The drawing under review shows one solid part. Ordinate dimensions are in mm from its lowest x, y, z. A direction names the side the tool comes from. Give positions to 0.01 mm unless a question says otherwise; leave off trailing zeros. Order: outer loops, then holes, each group sorted by start corner. A loop starts at its lowest first (then second) coordinate and runs counter-clockwise, first axis right, second up. Notation, with made-up numbers: (49.5, 20) -> (75.5, 20) arc R26 cw to (75.5, 49) -> close; hole circle Ø2 at (-30.5, 5.5). An arc over 180 degrees is marked (long way). One line per item, written item: value. Start each with the question number.
1) Tool access review of the marked faces 5, 6 and 7: name each direction out of +Z, -Z, +X, -X, +Y, -Y from which nothing blocks a thin tool from reaching the whole face with its end or side.
2) Consider section C-C (y = 13.5). State the section outline as (x, z) points.
3) For pin 1 (1 mm diameter, centred on x = 25, z = 20.5, fed in from +Y); pin 2 (6 mm diameter, centred on x = 14.5, z = 20.5, fed in from -Y), all flat-tipped, find the tip position at first contact; note any pin that passes through.
4) Consider section D-D (y = 25). State the section outline as (x, z) points.
5) Consider section A-A (z = 26.5). State the section outline as (x, y) points.
6) The part is to be moulded in two halves that separate along X. For the marked faces 1, 2, 3 and 4, say which applies: released by +X, released by -X, zero draft, split by the parting line, or undercut.
7) Wall thickness on line 1 along Z through (x, y) = (10, 7); line 2 along X through (y, z) = (26.5, 28.5); line 3 along Y through (x, z) = (20, 36): over which ranges is each line inside the solid? List them lowest first. Write a range as from..to.
8) Consider section B-B (x = 15). State the section outline as (y, z) points, plus the area to 3 significant figures.
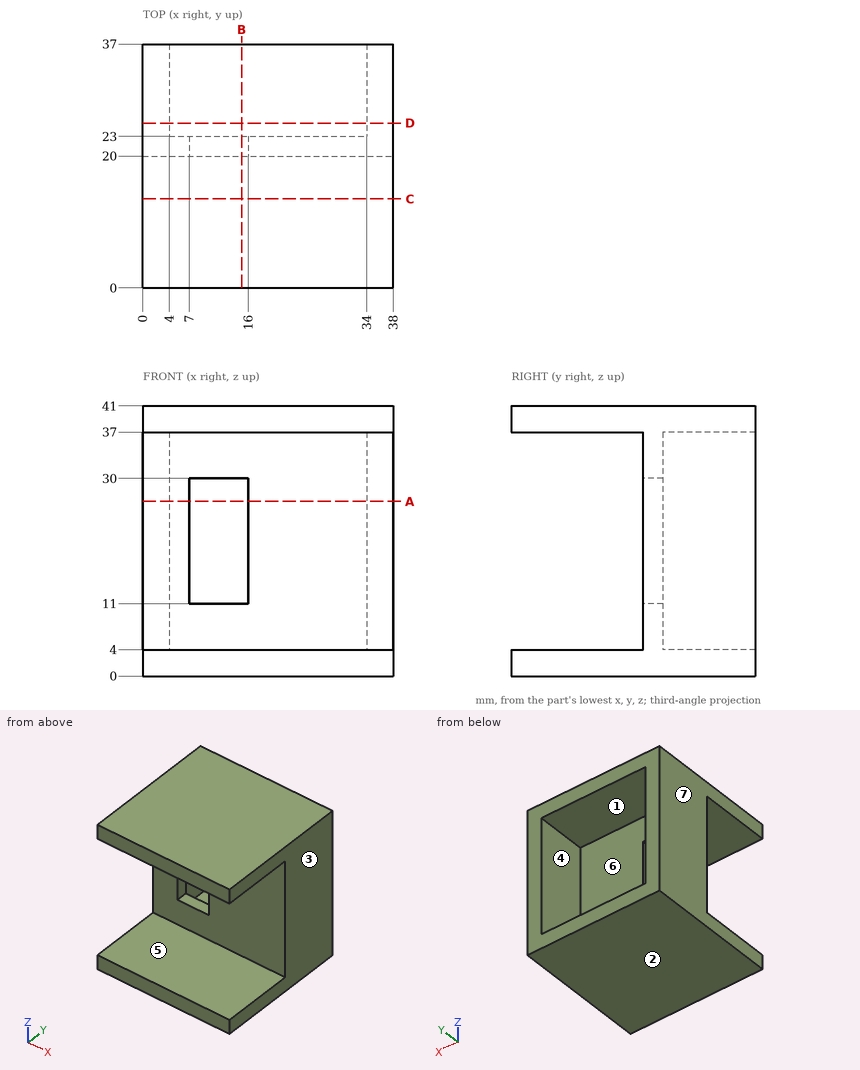
Checked values:
1. face 5: +X, -X, -Y
1. face 6: +Y
1. face 7: +Z, -Z, -X, +Y, -Y
2. outline: (0, 0) -> (38, 0) -> (38, 4) -> (0, 4) -> close; (0, 37) -> (38, 37) -> (38, 41) -> (0, 41) -> close
3. pin 1: stops at y = 23
3. pin 2: stops at y = 20
4. outline: (0, 0) -> (38, 0) -> (38, 41) -> (0, 41) -> close; hole (4, 4) -> (34, 4) -> (34, 37) -> (4, 37) -> close
5. outline: (0, 20) -> (7, 20) -> (7, 23) -> (4, 23) -> (4, 37) -> (0, 37) -> close; (16, 20) -> (38, 20) -> (38, 37) -> (34, 37) -> (34, 23) -> (16, 23) -> close
6. face 1: undercut
6. face 2: zero draft
6. face 3: released by +X
6. face 4: undercut
7. line 1: z = 0..4, 37..41
7. line 2: x = 0..4, 34..38
7. line 3: y = 20..23
8. outline: (0, 0) -> (37, 0) -> (37, 4) -> (23, 4) -> (23, 11) -> (20, 11) -> (20, 4) -> (0, 4) -> close; (0, 37) -> (20, 37) -> (20, 30) -> (23, 30) -> (23, 37) -> (37, 37) -> (37, 41) -> (0, 41) -> close
8. area: 338 mm^2
